```python
from build123d import *

# Parameters (mm, degrees)
SKETCH1_W           = 267.5
SKETCH1_H           = 536
SKETCH1_R           = 2.75
BOSS_EXTRUDE1_DEPTH = 8
CUT_EXTRUDE1_DEPTH  = 8
SKETCH3_R           = 1.864271291
SKETCH3_R_2         = 1.75
CUT_EXTRUDE2_DEPTH  = 10


with BuildPart() as part:
    # Sketch1 → Boss-Extrude1 (new body)
    with BuildSketch(Plane.XY):
        with Locations((-133.75, 0)):
            Rectangle(SKETCH1_W, SKETCH1_H)
        with Locations((-257.509341423, -143.000001745)):
            Circle(SKETCH1_R, mode=Mode.SUBTRACT)
        with Locations(Location((-257.5, 168, 0), (0, 0, 180))):
            Circle(SKETCH1_R, mode=Mode.SUBTRACT)
        with Locations(Location((-257.509341423, 143.000001745, 0), (0, 0, 180))):
            Circle(SKETCH1_R, mode=Mode.SUBTRACT)
        with Locations((-257.5, -168)):
            Circle(SKETCH1_R, mode=Mode.SUBTRACT)
    extrude(amount=BOSS_EXTRUDE1_DEPTH)

    # Sketch2 → Cut-Extrude1 (cut)
    with BuildSketch(Plane.XY.offset(8)):
        with BuildLine():
            Line((-159.5, 208), (160.5, 208))
            ThreePointArc((160.5, 208), (188.784271247, 196.284271247), (200.5, 168))
            Line((200.5, 168), (200.5, -132))
            ThreePointArc((200.5, -132), (188.784271247, -160.284271247), (160.5, -172))
            Line((160.5, -172), (-159.5, -172))
            ThreePointArc((-159.5, -172), (-187.784271247, -160.284271247), (-199.5, -132))
            Line((-199.5, -132), (-199.5, 168))
            ThreePointArc((-199.5, 168), (-187.784271247, 196.284271247), (-159.5, 208))
        make_face()
    extrude(amount=-CUT_EXTRUDE1_DEPTH, mode=Mode.SUBTRACT)

    # Sketch3 → Cut-Extrude2 (cut)
    with BuildSketch(Plane.XY.offset(8)):
        with Locations((-11.058771906, 215.5)):
            Circle(SKETCH3_R)
        with Locations((-159.5, 215.5)):
            Circle(SKETCH3_R_2)
        with Locations((-207, 168)):
            Circle(SKETCH3_R_2)
        with Locations((-207, 18)):
            Circle(SKETCH3_R_2)
        with Locations((-207, -132)):
            Circle(SKETCH3_R_2)
        with Locations((-159.5, -179.5)):
            Circle(SKETCH3_R_2)
        with Locations((-11.058771906, -179.5)):
            Circle(SKETCH3_R_2)
    extrude(amount=-CUT_EXTRUDE2_DEPTH, mode=Mode.SUBTRACT)


solid = part.part
```
CAD build for the part. Positions are in the model's coordinates, mm. A direction names the side the tool comes from. Give positions to 0.01 mm unless a question says otherwise; leave off trailing zeros. Loops run counter-clockwise (first coordinate to the right, second up) from the corner with the lowest first, then second, coordinate; pieces in that order, holes last. Notation, with made-up numbers: M -2,71.5 L 50,71.5 A29 ccw 50,99.5 Z; hole C -14,64 d10. An arc over 180 degrees is marked long. Use one line per item in the form item = value.
Item 1: Drill centre lines: probe 1 along X at (y, z) = (-179.5, 2.5); probe 2 along Y at (x, z) = (-159.5, 2); probe 3 along X at (y, z) = (168, 4.5). Where is each one in solid material? Low to high. Write a range as from..to.
Determined:
probe_1 = -267.5..-161.25, -157.75..-12.81, -9.31..0
probe_2 = -268..-181.25, -177.75..-172, 208..213.75, 217.25..268
probe_3 = -267.5..-260.25, -254.75..-208.75, -205.25..-199.5
Item 2: Slice it at B-B (x = -93). List the corners of the cut face in (y, z), plus the area to 3 significant figures.
Determined:
outline = M -268,0 L -172,0 L -172,8 L -268,8 Z; M 208,0 L 268,0 L 268,8 L 208,8 Z
area = 1,250 mm2
Item 3: Which spindle directions (+Z, -Z, +X, -X, +Y, -Y) get a long thin tool onto all of the face, cutting with end or side? Do faces 1 (the face through (-187.472, -160.594, 4.056)), 2 (the face through (-225, -56, 0)). Say none if no direction does.
Determined:
face_1 = +Z, -Z, +X
face_2 = -Z, +X, -X, +Y, -Y
Item 4: Two-plate mould, pull along Y, no slides. Class faces 3 (the face through (-225, -56, 8)), 4 (the face through (-188.094, 195.972, 4.056)): pulls with the +Y half, pulls with the -Y half, needs draft (parallel to the pull), parting line crosses it, or undercut.
Determined:
face_3 = needs draft
face_4 = undercut
Item 5: Flat gauge pin, fed straight in: pin 1 (2.5 mm diameter, centred on y = -18.5, z = 5.5, fed in from +X). Where does the tip first touch, or does it go through?
Determined:
pin_1 = -199.5
Item 6: Slice it at A-A (z = 6.5). Count the separate pieces of the cut face and the enclosed holes in it, plus the area to 3 significant figures.
Determined:
separate_pieces = 1
enclosed_holes = 11
area = 68,100 mm2
Item 7: Slice it at C-C (y = 135). List the corners of the cut face in (x, z), plus the area to 3 significant figures.
Determined:
outline = M -267.5,0 L -199.5,0 L -199.5,8 L -267.5,8 Z
area = 544 mm2
Item 8: Slice it at D-D (x = -183). List the corners of the cut face in (y, z), plus the area to 3 significant figures.
Determined:
outline = M -268,0 L -164.37,0 L -164.37,8 L -268,8 Z; M 200.37,0 L 268,0 L 268,8 L 200.37,8 Z
area = 1,370 mm2
